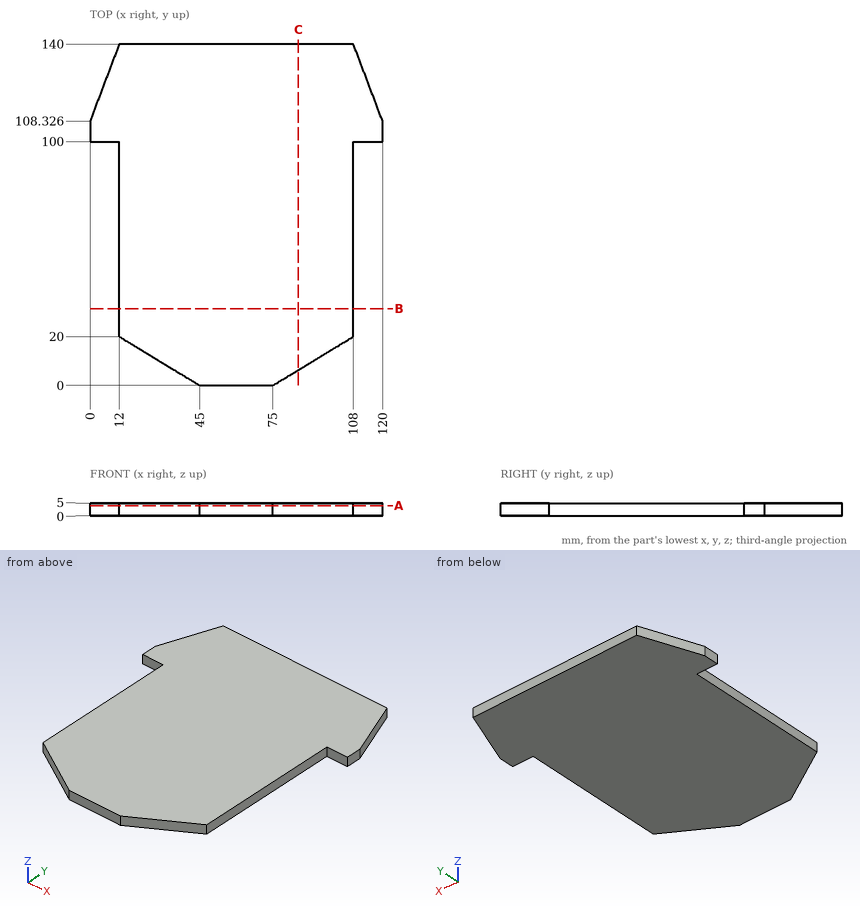
The figure shows three views and two pictorial views of one solid part (mm, origin at its lowest corner). Answer the questions. Round coordinates to 2 decimals unless told otherwise and drop trailing zeros. Order: outer loops, then holes, each group sorted by start corner. A loop starts at its lowest first (then second) coordinate and runs counter-clockwise, first axis right, second up. Notation, with made-up numbers: (86, 58.5) -> (110, 58.5) arc R17 cw to (110, 91.5) -> close; hole circle Ø1 at (3, 73). An arc over 180 degrees is marked (long way). One line per item, written item: value.
Item 1: Given P1, Ø1.5, axis at x = 8, z = 1.5, coming from the -Y side; P2, Ø2.5, axis at y = 54, z = 3, coming from the +X side; P3, Ø2.5, axis at y = 63.5, z = 2.5, coming from the -X side, each flat-ended and moving along its own axis, determine where each tip first touches the part or whether it passes through.
Taken from the geometry:
P1: stops at y = 100
P2: stops at x = 108
P3: stops at x = 12
Item 2: Find section B-B, the plane y = 31.5. Give the vertices of the cut face in (x, z).
Taken from the geometry:
outline: (12, 0) -> (108, 0) -> (108, 5) -> (12, 5) -> close
Item 3: Straight lines are drawn through the part: L1, parallel to X at y = 98.5, z = 3.15; L2, parallel to Y at x = 76, z = 2.65 (1 decimal); L3, parallel to X at y = 127.5, z = 2.6 (1 decimal). For each, find the intervals that lie inside material, in ascending order.
Taken from the geometry:
L1: x = 12 to 108
L2: y = 0.6 to 140
L3: x = 7.3 to 112.7
Item 4: Find section C-C, the plane x = 85.5. Give the vertices of the cut face in (y, z), then the cut area to 3 significant figures.
Taken from the geometry:
outline: (6.36, 0) -> (140, 0) -> (140, 5) -> (6.36, 5) -> close
area: 668 mm2
Item 5: Find section A-A, the plane z = 4.1. Give the vertices of the cut face in (x, y), then the cut area to 3 significant figures.
Taken from the geometry:
outline: (0, 100) -> (12, 100) -> (12, 20) -> (45, 0) -> (75, 0) -> (108, 20) -> (108, 100) -> (120, 100) -> (120, 108.33) -> (108, 140) -> (12, 140) -> (0, 108.33) -> close
area: 13,400 mm2
